Geometry: final body of the model. Coordinates: model frame, mm. A direction names the side the tool comes from. Give positions to 0.01 mm unless a question says otherwise; leave off trailing zeros. Loops run counter-clockwise (first coordinate to the right, second up) from the corner with the lowest first, then second, coordinate; pieces in that order, holes last. Notation, with made-up numbers: M -16,81.5 L 3,81.5 A11 cw 3,85.5 Z; hole C 81,-10 d10. An arc over 180 degrees is marked long. One line per question, with ' | ' between items. Start each with the question number.
from build123d import *

# Parameters (mm, degrees)
SKETCH1_W           = 139.7
SKETCH1_H           = 25.4
SKETCH1_R           = 6.35
BOSS_EXTRUDE1_DEPTH = 12.7
SKETCH4_W           = 45.72
SKETCH4_H           = 6.35
CUT_EXTRUDE1_DEPTH  = 13.335
FILLET1_R           = 3.175


with BuildPart() as part:
    # Sketch1 → Boss-Extrude1 (new body)
    with BuildSketch(Plane.XY):
        Rectangle(SKETCH1_W, SKETCH1_H)
        Circle(SKETCH1_R, mode=Mode.SUBTRACT)
    extrude(amount=BOSS_EXTRUDE1_DEPTH)

    # Sketch4 → Cut-Extrude1 (cut)
    with BuildSketch(Plane.XY.offset(12.7)):
        with Locations((-37.465, 0)):
            Rectangle(SKETCH4_W, SKETCH4_H)
        with Locations((37.465, 0)):
            Rectangle(SKETCH4_W, SKETCH4_H)
    extrude(amount=-CUT_EXTRUDE1_DEPTH, mode=Mode.SUBTRACT)

    # Fillet1
    fillet1_edges = [part.edges().sort_by_distance(p)[0] for p in [
        (-14.605, 3.175, 6.35),
        (-14.605, -3.175, 6.35),
        (-60.325, -3.175, 6.35),
        (-60.325, 3.175, 6.35),
        (14.605, 3.175, 6.35),
        (14.605, -3.175, 6.35),
        (60.325, -3.175, 6.35),
        (60.325, 3.175, 6.35),
    ]]
    fillet(fillet1_edges, radius=FILLET1_R - 0.0001)  # a hair under: the kernel refuses the full size


solid = part.part
Q1. Section A-A, the plane z = 10. Count the separate pieces of the cut face and the enclosed holes in it, plus the area to 3 significant figures.
Q2. Material intervals for L1, parallel to Y at x = 32, z = 12.25 (3 decimals); L2, parallel to Y at x = 0, z = 6.75; L3, parallel to X at y = -0.5, z = 10.5, sorted ascending.
Q3. Set-up query: faces 1 (the cylindrical face through (-15.51, 2.22, 6.26)), 2 (the flat face through (-1, 12.7, 6)). Return all of +Z, -Z, +X, -X, +Y, -Y with unobstructed straight access to the full face (end or side cutting, diameter ignored); none if empty.
Q4. Section B-B, the plane x = 35. Output: boundary loops of the cut face in (y, z) (3 decimals).
Q5. Section C-C, the plane x = 0. Output: boundary loops of the cut face in (y, z), plus the area to 3 significant figures.
Q6. Draft query along Y for faces 3 (the cylindrical face through (-15.56, -2.27, 6.26)), 4 (the cylindrical face through (-1.38, -6.2, 6.26)), 5 (the flat face through (-1, -12.7, 6)), 6 (the flat face through (69.85, 0, 6)). Return one class per face: released by +Y, released by -Y, zero draft, split by the parting line, or undercut.
Model answer:
1) separate pieces: 1 | enclosed holes: 3 | area: 2,860 mm^2
2) L1: y = -12.7 to -3.175, 3.175 to 12.7 | L2: y = -12.7 to -6.35, 6.35 to 12.7 | L3: x = -69.85 to -60.29, -14.64 to -6.33, 6.33 to 14.64, 60.29 to 69.85
3) face 1: +Z, -Z | face 2: +Z, -Z, +X, -X, +Y
4) outline: M -12.7,0 L -3.175,0 L -3.175,12.7 L -12.7,12.7 Z; M 3.175,0 L 12.7,0 L 12.7,12.7 L 3.175,12.7 Z
5) outline: M -12.7,0 L -6.35,0 L -6.35,12.7 L -12.7,12.7 Z; M 6.35,0 L 12.7,0 L 12.7,12.7 L 6.35,12.7 Z | area: 161 mm^2
6) face 3: undercut | face 4: undercut | face 5: released by -Y | face 6: zero draft
